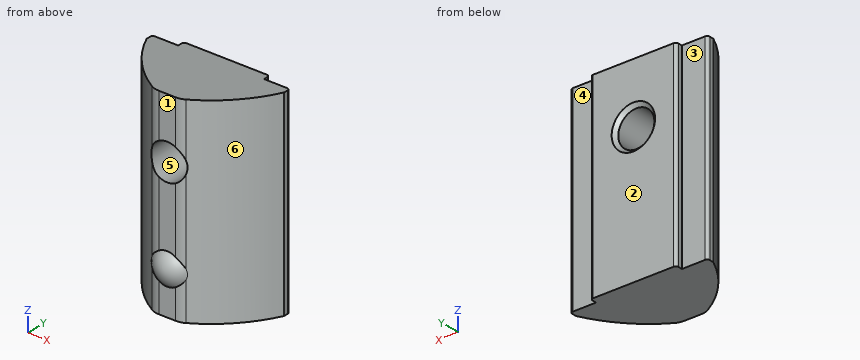
from build123d import *

# Parameters (mm, degrees)
EXTRUDE_1_DEPTH             = 11.5
FILLET_1_R                  = 0.3
FILLET_2_R                  = 2
HOLE_WIZARD_M53_D           = 4.2
HOLE_WIZARD_M53_CSINK_D     = 5.05
HOLE_WIZARD_M53_CSINK_ANGLE = 90


with BuildPart() as part:
    # Эскиз1 → Бобышка-Вытянуть1 (new body, symmetric)
    with BuildSketch(Plane.XY):
        with BuildLine():
            Line((-5, 0), (5, 0))
            Line((5, 0), (5, -0.8))
            Line((5, -0.8), (8, -0.8))
            Line((8, -0.8), (8, -1.6))
            ThreePointArc((8, -1.6), (5.309398779, -5.576969864), (1.5, -8.5))
            Line((1.5, -8.5), (-1.5, -8.5))
            ThreePointArc((-1.5, -8.5), (-5.309398779, -5.576969864), (-8, -1.6))
            Line((-8, -1.6), (-8, -0.8))
            Line((-8, -0.8), (-5, -0.8))
            Line((-5, -0.8), (-5, 0))
        make_face()
    extrude(amount=EXTRUDE_1_DEPTH, both=True)

    # Скругление1
    fillet_1_edges = [part.edges().sort_by_distance(p)[0] for p in [
        (8, -0.8, 0),
        (8, -1.6, 0),
        (-8, -1.6, 0),
        (-8, -0.8, 0),
        (-5, 0, 0),
        (5, 0, 0),
    ]]
    fillet(fillet_1_edges, radius=FILLET_1_R)

    # Скругление2
    fillet_2_edges = [part.edges().sort_by_distance(p)[0] for p in [
        (1.5, -8.5, 0),
        (-1.5, -8.5, 0),
    ]]
    fillet(fillet_2_edges, radius=FILLET_2_R)

    # Отверстие обработанное метчиком M53 (through all)
    with Locations(Plane(origin=(0, 0, 0), x_dir=(1, 0, 0), z_dir=(0, 1, 0))):
        with Locations((0, -4.5)):
            CounterSinkHole(HOLE_WIZARD_M53_D / 2, HOLE_WIZARD_M53_CSINK_D / 2, counter_sink_angle=HOLE_WIZARD_M53_CSINK_ANGLE)

    # Эскиз5 → Повернуть1 (revolve)
    with BuildSketch(Plane(origin=(0, 0, 0), x_dir=(0, 0, -1), z_dir=(1, 0, 0))):
        with BuildLine():
            Line((6.5, -4.3), (6.5, -9.3))
            ThreePointArc((6.5, -9.3), (4, -6.8), (6.5, -4.3))
        make_face()
    revolve(axis=Axis((0, -4.3, -6.5), (0, -1, 0)))


solid = part.part
Part model, mm, in its own coordinate system. Face numbers are marked on the shaded views. A direction names the side the tool comes from. Give positions to 0.01 mm unless a question says otherwise; leave off trailing zeros. Loops run counter-clockwise (first coordinate to the right, second up) from the corner with the lowest first, then second, coordinate; pieces in that order, holes last. Notation, with made-up numbers: M -30,38 L -26,38 A29 ccw -26,68 Z; hole C -6,-4 d1. An arc over 180 degrees is marked long. Put each result on its own line as item: value. Start each with the question number.
1) Flat gauge pins, fed straight in: pin 1 (1.6 mm diameter, centred on x = 0.5, z = -2.5, fed in from -Y); pin 2 (4 mm diameter, centred on y = -2, z = -9, fed in from +X); pin 3 (5 mm diameter, centred on x = -4, z = -5, fed in from -Y); pin 4 (2 mm diameter, centred on y = -5.5, z = -5.5, fed in from -X). Where does each tip first touch, or does it go through?
2) Pull direction X, two halves, no side cores. Call the marked faces 4, 5 and 6: +X half, -X half, draft (parallel to the pull), parting line (faces both ways), or undercut.
3) Probe probe 1 along Z at (x, y) = (0, -3.75); probe 2 along X at (y, z) = (-7.25, 6); probe 3 along Z at (x, y) = (0.5, -5.25). List the from-to ranges inside material, lowest first.
4) Saw through at D-D (z = -5.5). List the corners of the cut face in (x, y).
5) Saw through at A-A (x = 0). List the corners of the cut face in (y, z) (3 decimals).
6) 3-axis set-ups, long thin cutter, end or side, ignore diameter. For the marked faces 1, 2 and 3: which of +Z, -Z, +X, -X, +Y, -Y reach the whole face in a straight line?
7) Saw through at B-B (z = -1.75). List the corners of the cut face in (x, y), then the cut area to 3 significant figures.
Numbers:
1. pin 1: y = -8.5
1. pin 2: x = 8
1. pin 3: y = -8.56
1. pin 4: x = -6.23
2. face 4: draft
2. face 5: undercut
2. face 6: +X half
3. probe 1: -11.5 to 2.4, 6.6 to 11.5
3. probe 2: -3.45 to -1.47, 1.47 to 3.45
3. probe 3: -11.5 to 2.46, 6.54 to 11.5
4. outline: M -8,-1.53 A0.3 ccw -7.97,-1.66 A15 ccw -1.99,-8.22 A2 ccw -1.66,-8.38 A2.29 ccw 1.66,-8.38 A2 ccw 1.99,-8.22 A15 ccw 7.97,-1.66 A0.3 ccw 8,-1.53 L 8,-1.1 A0.3 ccw 7.7,-0.8 L 5,-0.8 L 5,-0.3 A0.3 ccw 4.7,0 L -4.7,0 A0.3 ccw -5,-0.3 L -5,-0.8 L -7.7,-0.8 A0.3 ccw -8,-1.1 Z
5. outline: M -8.5,-11.5 L 0,-11.5 L 0,1.975 L -0.425,2.4 L -8.5,2.4 L -8.5,-4.667 A2.5 ccw -8.5,-8.333 Z; M -8.5,6.6 L -0.425,6.6 L 0,7.025 L 0,11.5 L -8.5,11.5 Z
6. face 1: +Z, +X, -X, -Y
6. face 2: +Z, -Z, +X, -X, +Y
6. face 3: +Z, -Z, -X, +Y
7. outline: M -8,-1.53 A0.3 ccw -7.97,-1.66 A15 ccw -1.99,-8.22 A2 ccw -0.98,-8.5 L 0.98,-8.5 A2 ccw 1.99,-8.22 A15 ccw 7.97,-1.66 A0.3 ccw 8,-1.53 L 8,-1.1 A0.3 ccw 7.7,-0.8 L 5,-0.8 L 5,-0.3 A0.3 ccw 4.7,0 L -4.7,0 A0.3 ccw -5,-0.3 L -5,-0.8 L -7.7,-0.8 A0.3 ccw -8,-1.1 Z
7. area: 96.0 mm^2
